```python
from build123d import *

# Parameters (mm, degrees)
SKETCH_1_R      = 1
SKETCH_1_R_2    = 2
SKETCH_1_W      = 10
SKETCH_1_H      = 3
EXTRUDE_1_DEPTH = 3


with BuildPart() as part:
    # 草图1 → 凸台-拉伸1 (new body)
    with BuildSketch(Plane.XY):
        Polygon((-40, 17.5), (-40, 12.5), (-43, 12.5), (-43, 2.5), (-40, 2.5), (-40, -2.5), (-43, -2.5), (-43, -12.5), (-40, -12.5), (-40, -17.5), (-43, -17.5), (-43, -27.5), (-40, -27.5), (-40, -32.5), (40, -32.5), (40, -27.5), (43, -27.5), (43, -17.5), (40, -17.5), (40, -12.5), (43, -12.5), (43, -2.5), (40, -2.5), (40, 2.5), (43, 2.5), (43, 12.5), (40, 12.5), (40, 17.5), (43, 17.5), (43, 27.5), (40, 27.5), (40, 32.5), (-40, 32.5), (-40, 27.5), (-43, 27.5), (-43, 17.5), align=None)
        with Locations((-32.5, 16.5)):
            Circle(SKETCH_1_R, mode=Mode.SUBTRACT)
        with Locations(Location((32.5, 16.5, 0), (0, 0, 180))):
            Circle(SKETCH_1_R, mode=Mode.SUBTRACT)
        with Locations(Location((-32.5, -16.5, 0), (0, 0, 180))):
            Circle(SKETCH_1_R, mode=Mode.SUBTRACT)
        with Locations((32.5, -16.5)):
            Circle(SKETCH_1_R, mode=Mode.SUBTRACT)
        with Locations((0, 22.5)):
            Circle(SKETCH_1_R_2, mode=Mode.SUBTRACT)
        with Locations(Location((0, -22.5, 0), (0, 0, 180))):
            Circle(SKETCH_1_R_2, mode=Mode.SUBTRACT)
        with Locations((-10, 29)):
            Rectangle(SKETCH_1_W, SKETCH_1_H, mode=Mode.SUBTRACT)
        with Locations((-30, 29)):
            Rectangle(SKETCH_1_W, SKETCH_1_H, mode=Mode.SUBTRACT)
        with Locations((10, 29)):
            Rectangle(SKETCH_1_W, SKETCH_1_H, mode=Mode.SUBTRACT)
        with Locations((30, 29)):
            Rectangle(SKETCH_1_W, SKETCH_1_H, mode=Mode.SUBTRACT)
        with Locations((30, -29)):
            Rectangle(SKETCH_1_W, SKETCH_1_H, mode=Mode.SUBTRACT)
        with Locations((10, -29)):
            Rectangle(SKETCH_1_W, SKETCH_1_H, mode=Mode.SUBTRACT)
        with Locations((-10, -29)):
            Rectangle(SKETCH_1_W, SKETCH_1_H, mode=Mode.SUBTRACT)
        with Locations((-30, -29)):
            Rectangle(SKETCH_1_W, SKETCH_1_H, mode=Mode.SUBTRACT)
    extrude(amount=EXTRUDE_1_DEPTH)


solid = part.part
```
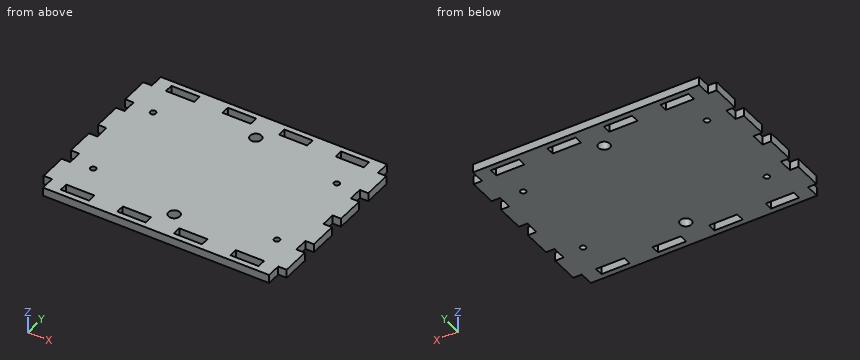
The model under review builds one solid part; all positions refer to its coordinate system, in mm. Give positions to 0.01 mm unless a question says otherwise; leave off trailing zeros. Write each loop counter-clockwise with the first axis right and the second up, starting at its lowest first coordinate (ties: lowest second). Pieces come first, ordered by that corner, then holes.
(1) To check wall thickness, follow L1, parallel to Y at x = 31, z = 1.55; L2, parallel to Y at x = 32.5, z = 0.7; L3, parallel to X at y = 28, z = 0.85. State the ranges of each line that lie inside material, in increasing order.
(2) Consider section C-C, the plane x = 27. Give the boundary of the cut face in (y, z), and give its area (3 significant figures).
(3) Consider section A-A, the plane x = -32.5. Give the boundary of the cut face in (y, z), and give its area (3 significant figures).
(4) Consider section B-B, the plane y = 22.5. Give the boundary of the cut face in (x, z).
(5) Consider section D-D, the plane y = -16.5. Give the boundary of the cut face in (x, z), and give its area (3 significant figures).
(6) For P1, Ø6.5, axis at x = 0, y = 22.5, coming from the +Z side; P2, Ø0.9, axis at x = 41, z = 1, coming from the +Y side; P3, Ø3.5, axis at x = 0, y = -22.5, coming from the -Z side; P4, Ø1.5, axis at y = 29, z = 1.5, coming from the -X side, all flat-tipped, find the tip position at first contact; note any pin that passes through.
Returned:
1. L1: y = -32.5 to -30.5, -27.5 to 27.5, 30.5 to 32.5
1. L2: y = -32.5 to -30.5, -27.5 to -17.5, -15.5 to 15.5, 17.5 to 27.5, 30.5 to 32.5
1. L3: x = -40 to -35, -25 to -15, -5 to 5, 15 to 25, 35 to 40
2. outline: (-32.5, 0) - (-30.5, 0) - (-30.5, 3) - (-32.5, 3) - close; (-27.5, 0) - (27.5, 0) - (27.5, 3) - (-27.5, 3) - close; (30.5, 0) - (32.5, 0) - (32.5, 3) - (30.5, 3) - close
2. area: 177 mm2
3. outline: (-32.5, 0) - (-30.5, 0) - (-30.5, 3) - (-32.5, 3) - close; (-27.5, 0) - (-17.5, 0) - (-17.5, 3) - (-27.5, 3) - close; (-15.5, 0) - (15.5, 0) - (15.5, 3) - (-15.5, 3) - close; (17.5, 0) - (27.5, 0) - (27.5, 3) - (17.5, 3) - close; (30.5, 0) - (32.5, 0) - (32.5, 3) - (30.5, 3) - close
3. area: 165 mm2
4. outline: (-43, 0) - (-2, 0) - (-2, 3) - (-43, 3) - close; (2, 0) - (43, 0) - (43, 3) - (2, 3) - close
5. outline: (-40, 0) - (-33.5, 0) - (-33.5, 3) - (-40, 3) - close; (-31.5, 0) - (31.5, 0) - (31.5, 3) - (-31.5, 3) - close; (33.5, 0) - (40, 0) - (40, 3) - (33.5, 3) - close
5. area: 228 mm2
6. P1: stops at z = 3
6. P2: stops at y = 27.5
6. P3: passes through
6. P4: stops at x = -40
